Autodesk Fusion 360 part; units mm, degrees
sketch "Sketch1" plane through (0, 0, 0) normal (0, 1, 0) x (1, 0, 0)
  line L0 (5, -5) -> (93, -5)
  arc A0 (93, -5) -> (93, 5) centre (93, 0) ccw
  line L1 (93, 5) -> (5, 5)
  arc A1 (5, 5) -> (5, -5) centre (5, 0) ccw
  line L2 (49, 5) -> (49, -5) construction
  line L3 (50, 0) -> (71, 0) construction
  line L4 (53, 2) -> (47, 2)
  arc A2 (47, 2) -> (47, -2) centre (47, 0) ccw
  line L5 (47, -2) -> (53, -2)
  arc A3 (53, -2) -> (53, 2) centre (53, 0) ccw
  line L6 (53, 0) -> (47, 0) construction
  line L7 (68, -2) -> (74, -2)
  arc A4 (74, -2) -> (74, 2) centre (74, 0) ccw
  line L8 (74, 2) -> (68, 2)
  arc A5 (68, 2) -> (68, -2) centre (68, 0) ccw
  line L9 (68, 0) -> (74, 0) construction
  point P0 (98, 0)
  point P1 (50, 0)
  point P2 (71, 0)
  point P3 (49, 0)
  dimension "d1" = 10
  dimension "d3" = 98
  dimension "d4" = 4
  dimension "d5" = 6
  dimension "d6" = 6
  dimension "d7" = 21
  dimension "d8" = 1
extrude "Extrude1" add sketch "Sketch1" along normal blind 3
Input: part model. Units: mm. Frame: model coordinates. A direction names the side the tool comes from. Coordinates: 2 decimals unless noted, no trailing zeros. Write each loop counter-clockwise with the first axis right and the second up, starting at its lowest first coordinate (ties: lowest second). Pieces come first, ordered by that corner, then holes. Notation, with made-up numbers: (55, 1.5) -> (65, 1.5) arc R18 cw to (65, 31.5) -> close; hole circle Ø9 at (-12.75, -20.75). An arc over 180 degrees is marked (long way). Write each question's results on one line, items separated by ' | '.
Item 1: Mould query, pull axis X, two halves, no side actions, for faces 3 (the cylindrical face through (0, 1, 0)), 4 (the flat face through (48.3, 0, -2.3)), 5 (the flat face through (50, 1, 2)), 6 (the cylindrical face through (55, 1, 0)). Classes: +X half, -X half, draft (parallel to the pull), parting line (faces both ways), or undercut.
Conclusion:
face 3: -X half | face 4: draft | face 5: undercut | face 6: undercut
Item 2: Section query C-C on y = 2.2. Return loops of the section in (x, z), plus the area to 3 significant figures.
Conclusion:
outline: (5, -5) -> (93, -5) arc R5 ccw to (93, 5) -> (5, 5) arc R5 ccw to start; hole (47, -2) -> (53, -2) arc R2 ccw to (53, 2) -> (47, 2) arc R2 ccw to start; hole (68, -2) -> (74, -2) arc R2 ccw to (74, 2) -> (68, 2) arc R2 ccw to start | area: 885 mm^2
Item 3: Section query D-D on z = 3.5. Return loops of the section in (x, y), plus the area to 3 significant figures.
Conclusion:
outline: (1.43, 0) -> (96.57, 0) -> (96.57, 3) -> (1.43, 3) -> close | area: 285 mm^2
Item 4: Section query B-B on z = -0.5. Return loops of the section in (x, y), plus the area to 3 significant figures.
Conclusion:
outline: (0.03, 0) -> (45.06, 0) -> (45.06, 3) -> (0.03, 3) -> close; (54.94, 0) -> (66.06, 0) -> (66.06, 3) -> (54.94, 3) -> close; (75.94, 0) -> (97.97, 0) -> (97.97, 3) -> (75.94, 3) -> close | area: 235 mm^2
Item 5: Material intervals for probe 1 along X at (y, z) = (2.95, 0.25); probe 2 along X at (y, z) = (0.45, 0.5); probe 3 along Z at (x, y) = (46, 0.45), sorted ascending.
Conclusion:
probe 1: x = 0.01 to 45.02, 54.98 to 66.02, 75.98 to 97.99 | probe 2: x = 0.03 to 45.06, 54.94 to 66.06, 75.94 to 97.97 | probe 3: z = -5 to -1.73, 1.73 to 5
Item 6: Section query A-A on x = 69. Return loops of the section in (y, z).
Conclusion:
outline: (0, -5) -> (3, -5) -> (3, -2) -> (0, -2) -> close; (0, 2) -> (3, 2) -> (3, 5) -> (0, 5) -> close
Item 7: Set-up query: faces 1 (the flat face through (48, 1, 5)), 2 (the flat face through (71, 1, 2)). Return all of +Z, -Z, +X, -X, +Y, -Y with unobstructed straight access to the full face (end or side cutting, diameter ignored); none if empty.
Conclusion:
face 1: +Z, +X, -X, +Y, -Y | face 2: +Y, -Y
Item 8: Pin query (flat end, axial travel): pin 1 Ø1.5 at (y, z) = (1, 2.5) entering from +X. Return the tip coordinate at first contact, or that it passes through.
Conclusion:
pin 1: stops at x = 97.68
